Verification items for the finished model (mm, model axes). Face numbers are marked on the shaded views. Give positions to 0.01 mm unless a question says otherwise; leave off trailing zeros. Write each loop counter-clockwise with the first axis right and the second up, starting at its lowest first coordinate (ties: lowest second). Pieces come first, ordered by that corner, then holes. Notation, with made-up numbers: (72.5, 58) -> (119.5, 58) arc R16 cw to (119.5, 69) -> close; hole circle Ø1 at (-7, -34). An arc over 180 degrees is marked (long way). Write item = value, one per line.
from build123d import *

# Parameters (mm, degrees)
F0_R      = 3.1
F1_DEPTH  = 88.12
F3_DEPTH  = 22.4
F5_DEPTH  = 62.8
F6_R      = 2.95
F7_DEPTH  = 62.8
F9_DEPTH  = 12.5
F10_R     = 1.5
F11_DEPTH = 7.9


with BuildPart() as f1:
    # F0 (on Front) → F1 (new body)
    with BuildSketch(Plane.XZ):
        Circle(F0_R)
    extrude(amount=F1_DEPTH)

    # F2 (on face) → F3 (cut)
    with BuildSketch(Plane.XZ.offset(88.12)):
        with BuildLine():
            ThreePointArc((3.1, 0), (0, 3.1), (-3.1, 0))
            Line((-3.1, 0), (3.1, 0))
        make_face()
    extrude(amount=-F3_DEPTH, mode=Mode.SUBTRACT)

    # F4 (on face) → F5 (cut)
    with BuildSketch(Plane(origin=(0, 0, 0), x_dir=(-1, 0, 0), z_dir=(0, 1, 0))):
        with BuildLine():
            ThreePointArc((3.1, 0), (0, 3.1), (-3.1, 0))
            Line((-3.1, 0), (3.1, 0))
        make_face()
    extrude(amount=-F5_DEPTH, mode=Mode.SUBTRACT)

    # F6 (on face) → F7 (cut)
    with BuildSketch(Plane(origin=(0, 0, 0), x_dir=(-1, 0, 0), z_dir=(0, 1, 0))):
        Circle(F6_R)
    extrude(amount=-F7_DEPTH, mode=Mode.SUBTRACT)

    # F8 (on Right) → F9 (cut, symmetric)
    with BuildSketch(Plane.YZ):
        Polygon((0, 0), (-18.3, 0), (-18.3, -0.55), (-9.9, -0.55), (-9.9, -1), (-4.1, -1), (-4.1, -1.4), (0, -1.4), align=None)
    extrude(amount=F9_DEPTH, both=True, mode=Mode.SUBTRACT)

    # F10 (on face) → F11 (join)
    with BuildSketch(Plane.XY):
        with Locations((0, -83.32)):
            Circle(F10_R)
    extrude(amount=-F11_DEPTH)


solid = f1.part
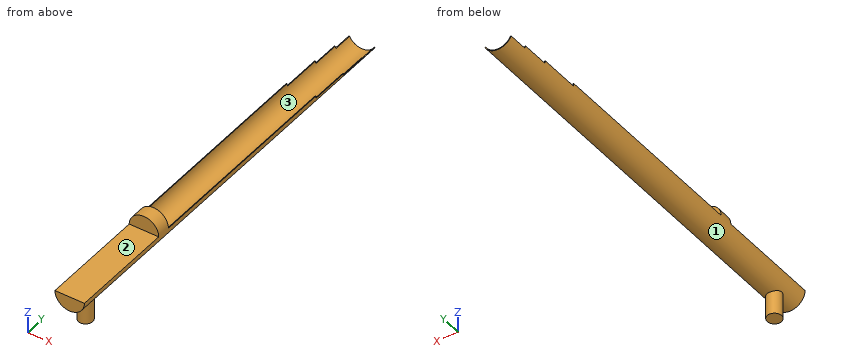
Item 1: Go/stop test with flat-tipped pins: P1, Ø1.5, axis at x = -2.5, y = -34, coming from the -Z side; P2, Ø3, axis at x = 2.5, y = -17, coming from the -Z side; P3, Ø3.5, axis at x = 1.5, z = 2, coming from the -Y side. Record where each tip stops, or that it passes through.
Response values:
P1 = -2.56
P2 = -2.93
P3 = -65.72
Item 2: Sectioned sample at D-D on z = 1. Record the cut outline in (x, y).
Response values:
outline = (-2.93, -65.72) -> (2.93, -65.72) -> (2.93, -62.8) -> (-2.93, -62.8) -> close
Item 3: Sectioned sample at B-B on y = -83.32. Record the cut outline in (x, z), then the cut area to 3 significant figures.
Response values:
outline = (-3.1, 0) arc R3.1 ccw to (-1.5, -2.71) -> (-1.5, -7.9) -> (1.5, -7.9) -> (1.5, -2.71) arc R3.1 ccw to (3.1, 0) -> close
area = 29.9 mm^2
Item 4: Material ranges on line 1 (Y direction, x = 1, z = -1.75); line 2 (Z direction, x = 1, y = -74); line 3 (Y direction, x = -1.25, z = 2), recorded low to high.
Response values:
line_1 = -88.12 to -62.8
line_2 = -2.93 to 0
line_3 = -65.72 to -62.8
Item 5: Sectioned sample at A-A on x = 0. Record the cut outline in (y, z), then the cut area to 3 significant figures.
Response values:
outline = (-88.12, -3.1) -> (-84.82, -3.1) -> (-84.82, -7.9) -> (-81.82, -7.9) -> (-81.82, -3.1) -> (0, -3.1) -> (0, -2.95) -> (-62.8, -2.95) -> (-62.8, 3.1) -> (-65.72, 3.1) -> (-65.72, 0) -> (-88.12, 0) -> close
area = 111 mm^2
Item 6: Sectioned sample at C-C on z = -5. Record the cut outline in (x, y), then the cut area to 3 significant figures.
Response values:
outline = circle Ø3 at (0, -83.32)
area = 7.07 mm^2
Item 7: Mould release check, pull along X, two halves, no side actions. Record for the marked faces 1, 2 and 3: +X half, -X half, draft (parallel to the pull), parting line (faces both ways), or undercut.
Response values:
face_1 = parting line
face_2 = draft
face_3 = undercut
